The model under review builds one solid part; all positions refer to its coordinate system, in mm. A direction names the side the tool comes from. Round coordinates to 2 decimals unless told otherwise and drop trailing zeros. Write each loop counter-clockwise with the first axis right and the second up, starting at its lowest first coordinate (ties: lowest second). Pieces come first, ordered by that corner, then holes. Notation, with made-up numbers: (-8.5, 55.25) -> (26.5, 55.25) arc R9 cw to (26.5, 60.25) -> close; hole circle Ø4 at (30, 60.25). An arc over 180 degrees is marked (long way). Return JSON: item names as keys, results as strings. Group by question number.
1. For line 1 along Z through (x, y) = (-27.5, 30); line 2 along Y through (x, z) = (-14.5, 7); line 3 along X through (y, z) = (14.5, 4), list the stretches that pass through material, from the lowest coordinate up. Write a range as from..to.
2. Tool access review of faces 1 (the flat face through (-22, 25, 15)), 2 (the flat face through (-15.16, 25.72, 7.4)): name each direction out of +Z, -Z, +X, -X, +Y, -Y from which nothing blocks a thin tool from reaching the whole face with its end or side.
3. Take a section at C-C, the plane z = 12. Write out the cut boundary in (x, y).
4. Take a section at A-A, the plane y = 17. Write out the cut boundary in (x, z), then the cut area to 3 significant figures.
5. Clearance check with flat-ended pins moving along their axes: P1, Ø1, axis at y = 10.5, z = 22, coming from the -X side; P2, Ø12, axis at x = -50.5, z = 28, coming from the -Y side; P3, Ø1, axis at x = -36.5, z = 27, coming from the -Y side; P4, Ø2, axis at x = -14.5, y = 30, coming from the -Z side. State where each tip first meets the part, or that it passes through.
6. Take a section at D-D, the plane x = -18. Write out the cut boundary in (y, z), then the cut area to 3 significant figures.
7. Take a section at B-B, the plane x = -39. Write out the cut boundary in (y, z), then the cut area to 3 significant figures.
Autodesk Inventor part; units mm, degrees
ref_plane "YZ Plane" through (0, 0, 0) normal (1, 0, 0) x (0, 1, 0)
ref_plane "XZ Plane" through (0, 0, 0) normal (0, 1, 0) x (-1, 0, 0)
ref_plane "XY Plane" through (0, 0, 0) normal (0, 0, 1) x (1, 0, 0)
sketch "Sketch1" plane through (0, 0, 0) normal (0, 0, 1) x (1, 0, 0)
  line L0 (-9.3066, 15.5847) -> (-20.8536, -4.4153)
  line L1 (-20.8536, -4.4153) -> (-43.9476, -4.4153)
  line L2 (-43.9476, -4.4153) -> (-55.4946, 15.5847)
  line L3 (-55.4946, 15.5847) -> (-43.9476, 35.5847)
  line L4 (-43.9476, 35.5847) -> (-20.8536, 35.5847)
  line L5 (-20.8536, 35.5847) -> (-9.3066, 15.5847)
  point P0 (0, 0)
  point P1 (-32.4006, 15.5847)
  dimension "d0" = 20
extrude "Extrusion1" add sketch "Sketch1" along normal blind 15
sketch "Sketch2" plane through (0, 0, 15) normal (0, 0, 1) x (1, 0, 0)
  circle A0 centre (-33.6983, 15.7961) radius 12.5
  point P0 (0, 0)
  dimension "d3" = 25
extrude "Extrusion2" add sketch "Sketch2" along normal blind 17
thread "Thread1"
properties part number "db screw 1"
Output:
{
 "1": {"line 1": "z = 0..15", "line 2": "y = 6.59..24.58", "line 3": "x = -54.87..-9.93"},
 "2": {"face 1": "+Z", "face 2": "+Z, -Z, +X, +Y"},
 "3": {"outline": "(-55.49, 15.58) -> (-43.95, -4.42) -> (-20.85, -4.42) -> (-9.31, 15.58) -> (-20.85, 35.58) -> (-43.95, 35.58) -> close"},
 "4": {"outline": "(-54.68, 0) -> (-10.12, 0) -> (-10.12, 15) -> (-21.26, 15) -> (-21.26, 32) -> (-46.14, 32) -> (-46.14, 15) -> (-54.68, 15) -> close", "area": "1,090 mm^2"},
 "5": {"P1": "stops at x = -45.24", "P2": "stops at y = 9.51", "P3": "stops at y = 3.51", "P4": "passes through"},
 "6": {"outline": "(0.53, 0) -> (30.64, 0) -> (30.64, 15) -> (0.53, 15) -> close", "area": "452 mm^2"},
 "7": {"outline": "(-4.42, 0) -> (35.58, 0) -> (35.58, 15) -> (27.12, 15) -> (27.12, 32) -> (4.48, 32) -> (4.48, 15) -> (-4.42, 15) -> close", "area": "985 mm^2"}
}
